```python
from build123d import *

# Parameters (mm, degrees)
SKETCH1_W           = 33
SKETCH1_H           = 31.85
SKETCH1_R           = 1.1
SKETCH1_W_2         = 12
SKETCH1_H_2         = 3
BOSS_EXTRUDE1_DEPTH = 2
SKETCH2_R           = 2.1
SKETCH2_R_2         = 1.1
BOSS_EXTRUDE2_DEPTH = 2.3
SKETCH3_W           = 33
SKETCH3_H           = 31.85
SKETCH3_W_2         = 29
SKETCH3_H_2         = 27.85
BOSS_EXTRUDE3_DEPTH = 2


with BuildPart() as part:
    # Sketch1 → Boss-Extrude1 (new body)
    with BuildSketch(Plane.XY):
        Rectangle(SKETCH1_W, SKETCH1_H)
        with Locations((-12.05, 11.575)):
            Circle(SKETCH1_R, mode=Mode.SUBTRACT)
        with Locations((12.05, 11.575)):
            Circle(SKETCH1_R, mode=Mode.SUBTRACT)
        with Locations((-12.05, -11.925)):
            Circle(SKETCH1_R, mode=Mode.SUBTRACT)
        with Locations((12.05, -11.925)):
            Circle(SKETCH1_R, mode=Mode.SUBTRACT)
        with Locations((0, -12.425)):
            Rectangle(SKETCH1_W_2, SKETCH1_H_2, mode=Mode.SUBTRACT)
    extrude(amount=BOSS_EXTRUDE1_DEPTH)

    # Sketch2 → Boss-Extrude2 (add)
    # profile 1 of 4: a face of its own
    with BuildSketch(Plane.XY.offset(2)):
        with Locations((-12.05, 11.575)):
            Circle(SKETCH2_R)
        with Locations((-12.05, 11.575)):
            Circle(SKETCH2_R_2, mode=Mode.SUBTRACT)
    # profile 2 of 4: a face of its own
    with BuildSketch(Plane.XY.offset(2)):
        with Locations((-12.05, -11.925)):
            Circle(SKETCH2_R)
        with Locations((-12.05, -11.925)):
            Circle(SKETCH2_R_2, mode=Mode.SUBTRACT)
    # profile 3 of 4: a face of its own
    with BuildSketch(Plane.XY.offset(2)):
        with Locations((12.05, -11.925)):
            Circle(SKETCH2_R)
        with Locations((12.05, -11.925)):
            Circle(SKETCH2_R_2, mode=Mode.SUBTRACT)
    # profile 4 of 4: a face of its own
    with BuildSketch(Plane.XY.offset(2)):
        with Locations((12.05, 11.575)):
            Circle(SKETCH2_R)
        with Locations((12.05, 11.575)):
            Circle(SKETCH2_R_2, mode=Mode.SUBTRACT)
    extrude(amount=BOSS_EXTRUDE2_DEPTH)

    # Sketch3 → Boss-Extrude3 (add)
    with BuildSketch(Plane.XY.offset(2)):
        Rectangle(SKETCH3_W, SKETCH3_H)
        Rectangle(SKETCH3_W_2, SKETCH3_H_2, mode=Mode.SUBTRACT)
    extrude(amount=BOSS_EXTRUDE3_DEPTH)


solid = part.part
```
Model file for the job. Use its own axes, mm. A direction names the side the tool comes from. Give positions to 0.01 mm unless a question says otherwise; leave off trailing zeros. Write each loop counter-clockwise with the first axis right and the second up, starting at its lowest first coordinate (ties: lowest second). Pieces come first, ordered by that corner, then holes. Notation, with made-up numbers: M 32,34 L 66,34 A30 cw 66,73 Z; hole C -30.75,68.25 d11. An arc over 180 degrees is marked long. Use a Markdown table: item, result.
1) Drill centre lines: line 1 (Y direction, x = 12.05, z = 2.2) (3 decimals); line 2 (X direction, y = 11.5, z = 0.65); line 3 (X direction, y = -12, z = 3.5). Where is each one in solid material? Low to high. Write a range as from..to.
Responses:
| item | result |
|---|---|
| line 1 | y = -15.925..-13.025, -10.825..-9.825, 9.475..10.475, 12.675..13.675, 13.925..15.925 |
| line 2 | x = -16.5..-13.15, -10.95..10.95, 13.15..16.5 |
| line 3 | x = -16.5..-14.5, -14.15..-13.15, -10.95..-9.95, 9.95..10.95, 13.15..14.15, 14.5..16.5 |
2) Pull direction X, two halves, no side cores. Call faces 4 (the cylindrical face through (-12.193, 12.666, 2.12)), 5 (the flat face through (-16.5, 0, 2)), 6 (the flat face through (0, -15.925, 2)): +X half, -X half, draft (parallel to the pull), parting line (faces both ways), or undercut.
Responses:
| item | result |
|---|---|
| face 4 | undercut |
| face 5 | -X half |
| face 6 | draft |
3) Cut at A-A (x = 12.05). List the corners of the cut face in (y, z) (3 decimals).
Responses:
| item | result |
|---|---|
| outline | M -15.925,0 L -13.025,0 L -13.025,4.3 L -14.025,4.3 L -14.025,4 L -15.925,4 Z; M -10.825,0 L 10.475,0 L 10.475,4.3 L 9.475,4.3 L 9.475,2 L -9.825,2 L -9.825,4.3 L -10.825,4.3 Z; M 12.675,0 L 15.925,0 L 15.925,4 L 13.925,4 L 13.925,2 L 13.675,2 L 13.675,4.3 L 12.675,4.3 Z |
4) Cut at D-D (y = -2). List the corners of the cut face in (x, z), and give its area (3 significant figures).
Responses:
| item | result |
|---|---|
| outline | M -16.5,0 L 16.5,0 L 16.5,4 L 14.5,4 L 14.5,2 L -14.5,2 L -14.5,4 L -16.5,4 Z |
| area | 74.0 mm2 |
5) Tool access for faces 1 (the flat face through (-14.5, 0, 3)), 2 (the flat face through (13, 10.7, 4.3)), 3 (the flat face through (6, -12, 1)): list every direction of +Z, -Z, +X, -X, +Y, -Y with a clear straight run to the whole face (end or side of a thin tool).
Responses:
| item | result |
|---|---|
| face 1 | +Z |
| face 2 | +Z, +X, -X, +Y, -Y |
| face 3 | +Z, -Z |
6) Pin check, flat tips, straight feed: pin 1 (4 mm diameter, centred on x = -5, y = -6.5, fed in from +Z); pin 2 (9.5 mm diameter, centred on x = -7.5, y = 8, fed in from +Z). Stop position of each tip, or through.
Responses:
| item | result |
|---|---|
| pin 1 | stops at z = 2 |
| pin 2 | stops at z = 4.3 |
7) Cut at C-C (x = 1.5). List the corners of the cut face in (y, z) (3 decimals).
Responses:
| item | result |
|---|---|
| outline | M -15.925,0 L -13.925,0 L -13.925,4 L -15.925,4 Z; M -10.925,0 L 15.925,0 L 15.925,4 L 13.925,4 L 13.925,2 L -10.925,2 Z |
8) Cut at B-B (z = 2.9). List the corners of the cut face in (x, y) (3 decimals).
Responses:
| item | result |
|---|---|
| outline | M -16.5,-15.925 L 16.5,-15.925 L 16.5,15.925 L -16.5,15.925 Z; C -12.05,11.575 d4.2; C 12.05,11.575 d4.2; hole M -14.5,-13.925 L -12.69,-13.925 A2.1 cw long -11.41,-13.925 L 11.41,-13.925 A2.1 cw long 12.69,-13.925 L 14.5,-13.925 L 14.5,13.925 L -14.5,13.925 Z; hole C -12.05,-11.925 d2.2; hole C -12.05,11.575 d2.2; hole C 12.05,-11.925 d2.2; hole C 12.05,11.575 d2.2 |
